Work out the finished part from the listing and answer in its coordinate system (mm). A direction names the side the tool comes from. Round coordinates to 2 decimals unless told otherwise and drop trailing zeros. Order: outer loops, then holes, each group sorted by start corner. A loop starts at its lowest first (then second) coordinate and runs counter-clockwise, first axis right, second up. Notation, with made-up numbers: M 1,-1.5 L 23,-1.5 A24 cw 23,23.5 Z; hole C 82,-34 d2. An arc over 180 degrees is marked long. Return JSON: item names as keys, results as strings.
Autodesk Inventor part; units mm, degrees
ref_plane "YZ Plane" through (0, 0, 0) normal (1, 0, 0) x (0, 1, 0)
ref_plane "XZ Plane" through (0, 0, 0) normal (0, 1, 0) x (-1, 0, 0)
ref_plane "XY Plane" through (0, 0, 0) normal (0, 0, 1) x (1, 0, 0)
sketch "Sketch1" plane through (0, 0, 0) normal (0, 0, 1) x (1, 0, 0)
  line L0 (17.9, -19.1) -> (17.9, 19.1)
  line L1 (15.9, 21.1) -> (-15.9, 21.1)
  line L2 (-17.9, 19.1) -> (-17.9, -19.1)
  line L3 (-15.9, -21.1) -> (-10.5924, -21.1)
  line L4 (17.9, -21.1) -> (-17.9, 21.1) construction
  line L5 (17.9, 21.1) -> (-17.9, -21.1) construction
  line L6 (-7.4, -17.4) -> (7.4, -17.4)
  line L7 (-7.4, -17.4) -> (-8.833, -20.051)
  line L8 (7.4, -17.4) -> (8.833, -20.051)
  line L9 (10.5924, -21.1) -> (15.9, -21.1)
  line L10 (-9.4, -21.1) -> (9.4, -21.1)
  arc A0 (-15.9, 21.1) -> (-17.9, 19.1) centre (-15.9, 19.1) ccw
  arc A1 (17.9, 19.1) -> (15.9, 21.1) centre (15.9, 19.1) ccw
  arc A2 (15.9, -21.1) -> (17.9, -19.1) centre (15.9, -19.1) ccw
  arc A3 (8.833, -20.051) -> (10.5924, -21.1) centre (10.5924, -19.1) ccw
  arc A4 (-10.5924, -21.1) -> (-8.833, -20.051) centre (-10.5924, -19.1) ccw
  arc A5 (-17.9, -19.1) -> (-15.9, -21.1) centre (-15.9, -19.1) ccw
  point P0 (0, 0)
  dimension "d0" = 35.8
  dimension "d1" = 42.2
  dimension "d2" = 38.5
  dimension "d3" = 10.5
  dimension "d4" = 10.5
  dimension "d5" = 8.5
  dimension "d6" = 8.5
  dimension "d7" = 2
extrude "Extrusion1" add sketch "Sketch1" along normal blind 1.8
sketch "Sketch2" plane through (0, 0, 1.8) normal (0, 0, 1) x (1, 0, 0)
  line L0 (-15.85, 15.1) -> (15.85, 15.1)
  line L1 (15.85, 15.1) -> (15.85, 17.6)
  line L2 (15.85, 17.6) -> (-15.85, 17.6)
  line L3 (-15.85, 17.6) -> (-15.85, 15.1)
  line L4 (-15.85, 15.1) -> (15.85, 17.6) construction
  line L5 (15.85, 15.1) -> (-15.85, 17.6) construction
  line L6 (15.9, 21.1) -> (-15.9, 21.1)
  point P0 (0, 0)
  point P1 (0, 16.35)
  point P2 (0, 16.35)
  point P3 (15.85, 16.35)
  point P4 (-15.85, 16.35)
  dimension "d10" = 2.5
  dimension "d11" = 6
  dimension "d12" = 31.7
extrude "Extrusion2" add sketch "Sketch2" along normal blind 1
fillet "Fillet1" radius 1 2 edges at (0, 17.6, 2.8) (0, 15.1, 2.8)
sketch "Sketch3" plane through (0, 0, 1.8) normal (0, 0, 1) x (1, 0, 0)
  line L0 (-12.9, 19.1) -> (12.9, 19.1)
  line L1 (13.9, 18.1) -> (13.9, -13.2)
  line L2 (12.9, -14.2) -> (-12.9, -14.2)
  line L3 (-13.9, -13.2) -> (-13.9, 18.1)
  line L4 (15.9, 21.1) -> (-15.9, 21.1)
  line L5 (-13.9, 2.9131) -> (-17.9, 2.9131)
  line L6 (-17.9, 19.1) -> (-17.9, -19.1)
  line L7 (13.9, 2.9131) -> (17.9, 2.9131)
  line L8 (17.9, -19.1) -> (17.9, 19.1)
  arc A0 (-12.9, 19.1) -> (-13.9, 18.1) centre (-12.9, 18.1) ccw
  arc A1 (13.9, 18.1) -> (12.9, 19.1) centre (12.9, 18.1) ccw
  arc A2 (12.9, -14.2) -> (13.9, -13.2) centre (12.9, -13.2) ccw
  arc A3 (-13.9, -13.2) -> (-12.9, -14.2) centre (-12.9, -13.2) ccw
  point P0 (0, 0)
  point P1 (13.9, -14.2)
  point P2 (13.9, 19.1)
  point P3 (-13.9, -14.2)
  dimension "d16" = 27.8
  dimension "d17" = 33.3
  dimension "d18" = 2
  dimension "d19" = 1
extrude "Extrusion3" add sketch "Sketch3" along normal blind 3.7
sketch "Sketch4" plane through (0, 0, 0) normal (0, 0, -1) x (-1, 0, 0)
  line L0 (-17.9, -19.1) -> (-17.9, 19.1)
  line L1 (17.9, 19.1) -> (17.9, -19.1)
  line L2 (-17.9, 6.6) -> (17.9, 6.6)
  line L3 (17.9, 6.6) -> (17.9, 4.1)
  line L4 (17.9, 4.1) -> (-17.9, 4.1)
  line L5 (-17.9, 4.1) -> (-17.9, 6.6)
  line L6 (-15.9, 21.1) -> (15.9, 21.1)
  point P0 (0, 0)
  dimension "d22" = 2.5
  dimension "d23" = 17
extrude "Extrusion4" add sketch "Sketch4" along normal blind 1
fillet "Fillet2" radius 1 2 edges at (0, 6.6, -1) (0, 4.1, -1)
sketch "Sketch5" plane through (0, 0, 0) normal (0, 0, -1) x (-1, 0, 0)
  line L0 (-14.8, 8.9) -> (14.8, 8.9)
  line L1 (15.8, 7.9) -> (15.8, -0.1)
  line L2 (14.8, -1.1) -> (-14.8, -1.1)
  line L3 (-15.8, -0.1) -> (-15.8, 7.9)
  line L4 (-15.9, 21.1) -> (15.9, 21.1)
  line L5 (-17.9, 6.6) -> (-17.9, 19.1)
  line L6 (17.9, 4.1) -> (17.9, -19.1)
  arc A0 (-15.8, -0.1) -> (-14.8, -1.1) centre (-14.8, -0.1) ccw
  arc A1 (-14.8, 8.9) -> (-15.8, 7.9) centre (-14.8, 7.9) ccw
  arc A2 (15.8, 7.9) -> (14.8, 8.9) centre (14.8, 7.9) ccw
  arc A3 (14.8, -1.1) -> (15.8, -0.1) centre (14.8, -0.1) ccw
  point P0 (0, 0)
  point P1 (0, 8.9)
  dimension "d27" = 22.2
  dimension "d28" = 2.1
  dimension "d29" = 10
  dimension "d30" = 2.1
  dimension "d31" = 1
extrude "Extrusion5" add sketch "Sketch5" along normal blind 26.3
sketch "Sketch6" plane through (0, 0, 0) normal (0, 0, -1) x (-1, 0, 0)
  line L0 (-5, 16.9799) -> (5, 16.9799)
  line L1 (5, 16.9799) -> (5, 8.9)
  line L2 (5, 8.9) -> (-5, 8.9)
  line L3 (-5, 8.9) -> (-5, 16.9799)
  line L4 (14.8, 8.9) -> (-14.8, 8.9)
  line L5 (5, 16.9799) -> (17.9, 16.9799)
  line L6 (17.9, 19.1) -> (17.9, 6.6)
  line L7 (-5, 16.9799) -> (-17.9, 16.9799)
  line L8 (-17.9, -19.1) -> (-17.9, 19.1)
  point P0 (0, 0)
  point P1 (-5, 12.94)
  dimension "d34" = 10
extrude "Extrusion6" cut sketch "Sketch6" against normal blind 4.5
sketch "Sketch7" plane through (-14.8, 8.9, -26.3) normal (0, 1, 0) x (1, 0, 0)
  line L0 (9.8, -30.8) -> (19.8, -30.8)
  line L1 (14.8, -30.8) -> (14.8, -11.8)
  line L2 (8.8, -11.8) -> (20.8, -11.8)
  line L3 (20.8, -11.8) -> (20.8, -10.8)
  line L4 (20.8, -10.8) -> (8.8, -10.8)
  line L5 (8.8, -10.8) -> (8.8, -11.8)
  line L6 (20.8, -11.8) -> (20.8, -13.8)
  line L7 (20.8, -13.8) -> (19.8, -13.8)
  line L8 (19.8, -13.8) -> (19.8, -11.8)
  line L9 (8.8, -11.8) -> (8.8, -13.8)
  line L10 (8.8, -13.8) -> (9.8, -13.8)
  line L11 (9.8, -13.8) -> (9.8, -11.8)
  point P0 (14.8, -26.3)
  dimension "d37" = 19
  dimension "d38" = 12
  dimension "d39" = 1
  dimension "d40" = 1
  dimension "d41" = 2
extrude "Extrusion7" add sketch "Sketch7" along normal blind 2
sketch "Sketch8" plane through (-14.8, 10.9, -26.3) normal (0, 1, 0) x (1, 0, 0)
  line L0 (9.8, -11.8) -> (19.8, -11.8)
  line L1 (20.8, -13.8) -> (20.8, -10.8)
  line L2 (19.8, -11.8) -> (20.8, -11.8)
  line L3 (20.8, -11.8) -> (20.8, -13.8)
  line L4 (20.8, -13.8) -> (19.8, -13.8)
  line L5 (19.8, -13.8) -> (19.8, -11.8)
  line L6 (9.8, -11.8) -> (9.8, -13.8)
  line L7 (8.8, -13.8) -> (8.8, -10.8)
  line L8 (9.8, -11.8) -> (8.8, -11.8)
  line L9 (8.8, -11.8) -> (8.8, -13.8)
  line L10 (8.8, -13.8) -> (9.8, -13.8)
  line L11 (9.8, -13.8) -> (9.8, -11.8)
  point P0 (14.8, -26.3)
extrude "Extrusion8" add sketch "Sketch8" along normal blind 2
sketch "Sketch9" plane through (5, 8.9, -14.5) normal (-1, 0, 0) x (0, 0, 1)
  line L0 (0, 2) -> (0, 4)
  line L1 (2, 0) -> (2, 4)
  line L2 (0, 4) -> (2, 4)
  line L3 (2, 4) -> (2, 2)
  line L4 (2, 2) -> (0, 2)
  line L5 (0, 2) -> (0, 4)
  point P0 (14.5, -8.9)
extrude "Extrusion9" add sketch "Sketch9" along normal blind 0.5
chamfer "Chamfer1" distance 2 angle 35 1 edges at (4.5, 12.9, -13.5) measured on face at (4.5, 11.5667, -13.8333)
mirror "Mirror1" about plane through (0, 0, 0) normal (1, 0, 0) of "Extrusion9", "Chamfer1"
sketch "Sketch10" plane through (0, 0, 4.5) normal (0, 0, -1) x (-1, 0, 0)
  line L0 (-4.5, 9.9) -> (4.5, 9.9)
  line L1 (5, 10.4) -> (5, 12)
  line L2 (4.5, 12.5) -> (-4.5, 12.5)
  line L3 (-5, 12) -> (-5, 10.4)
  line L4 (5, 8.9) -> (-5, 8.9)
  line L5 (-5, 8.9) -> (-5, 16.9799)
  arc A0 (-5, 10.4) -> (-4.5, 9.9) centre (-4.5, 10.4) ccw
  arc A1 (-4.5, 12.5) -> (-5, 12) centre (-4.5, 12) ccw
  arc A2 (5, 12) -> (4.5, 12.5) centre (4.5, 12) ccw
  arc A3 (4.5, 9.9) -> (5, 10.4) centre (4.5, 10.4) ccw
  point P0 (0, 0)
  point P1 (-5, 11.2)
  dimension "d51" = 1
  dimension "d52" = 10
  dimension "d53" = 0.5
  dimension "d54" = 2.6
extrude "Extrusion10" cut sketch "Sketch10" against normal blind 2
properties part number "PS2 USB C PD Mount"
Item 1: Consider line 1 along Z through (x, y) = (4, 9); line 2 along Z through (x, y) = (-14.5, -15); line 3 along X through (y, z) = (4, -14). Determine where each line is inside the solid, lowest interval first. Write a range as [from, to].
Output:
{"line 1": "z = [-15.5, -14.5], [4.5, 5.5]", "line 2": "z = [0, 1.8]", "line 3": "x = [-15.8, 15.8]"}
Item 2: The mould has two halves that part along X. Classify faces 4 (the flat face through (17.9, 0, 1)), 5 (the flat face through (0.1, 9.3, 4.5)), 6 (the cylindrical face through (16.865, 4.385, -0.699)): pulls with the +X half, pulls with the -X half, needs draft (parallel to the pull), parting line crosses it, or undercut.
Output:
{"face 4": "pulls with the +X half", "face 5": "undercut", "face 6": "needs draft"}
Item 3: Find section C-C (z = -23). Determine the outline of the cut face in (x, y), plus the area to 3 significant figures.
Output:
{"outline": "M -15.8,-0.1 A1 ccw -14.8,-1.1 L 14.8,-1.1 A1 ccw 15.8,-0.1 L 15.8,7.9 A1 ccw 14.8,8.9 L -14.8,8.9 A1 ccw -15.8,7.9 Z", "area": "315 mm^2"}
Item 4: Each of these flat-tipped pins is pushed along its axis until it touches: pin 1 (1.5 mm diameter, centred on x = -2.5, y = -10, fed in from -Z); pin 2 (10 mm diameter, centred on x = -8, z = -22.5, fed in from -Y); pin 3 (1.1 mm diameter, centred on x = 0.5, z = 5, fed in from +Y); pin 4 (8 mm diameter, centred on y = -15.5, z = -4.5, fed in from +X). Where does it stop, or does it pass through?
Output:
{"pin 1": "stops at z = 0", "pin 2": "stops at y = -1.1", "pin 3": "stops at y = 19.1", "pin 4": "passes through"}
Item 5: Which of the six approach directions +Z, -Z, +X, -X, +Y, -Y give full straight-line access (tool end or side, diameter ignored) to faces 1 (the cylindrical face through (14.861, 17.299, 2.515)), 2 (the cylindrical face through (15.515, 8.599, -12.966)), 3 (the flat face through (-5, 13, 2))?
Output:
{"face 1": "+Z, +X, +Y", "face 2": "-Z, +X, +Y", "face 3": "none"}
Item 6: Find section A-A (x = -2). Determine the outline of the cut face in (y, z), plus the area to 3 significant figures.
Output:
{"outline": "M -17.4,0 L -1.1,0 L -1.1,-26.3 L 8.9,-26.3 L 8.9,-15.5 L 10.9,-15.5 L 10.9,-14.5 L 8.9,-14.5 L 8.9,4.5 L 9.9,4.5 L 9.9,5.5 L -14.2,5.5 L -14.2,1.8 L -17.4,1.8 Z; M 12.5,4.5 L 16.98,4.5 L 16.98,0 L 21.1,0 L 21.1,1.8 L 19.1,1.8 L 19.1,5.5 L 12.5,5.5 Z", "area": "419 mm^2"}
Item 7: Find section B-B (y = 2). Determine the outline of the cut face in (x, z), plus the area to 3 significant figures.
Output:
{"outline": "M -17.9,0 L -15.8,0 L -15.8,-26.3 L 15.8,-26.3 L 15.8,0 L 17.9,0 L 17.9,1.8 L 13.9,1.8 L 13.9,5.5 L -13.9,5.5 L -13.9,1.8 L -17.9,1.8 Z", "area": "998 mm^2"}
Item 8: Find section D-D (x = -9.5). Determine the outline of the cut face in (y, z).
Output:
{"outline": "M -20.78,0 L -1.1,0 L -1.1,-26.3 L 8.9,-26.3 L 8.9,0 L 21.1,0 L 21.1,1.8 L 19.1,1.8 L 19.1,5.5 L -14.2,5.5 L -14.2,1.8 L -20.78,1.8 Z"}
